Model file for the job. Use its own axes, mm. A direction names the side the tool comes from. Coordinates: 2 decimals unless noted, no trailing zeros. Write each loop counter-clockwise with the first axis right and the second up, starting at its lowest first coordinate (ties: lowest second). Pieces come first, ordered by that corner, then holes.
Q1. Pin check, flat tips, straight feed: P1, Ø2, axis at x = -142, y = 57, coming from the +Z side; P2, Ø16.5, axis at x = -127.5, z = 39.5, coming from the +Y side; P3, Ø16, axis at x = 251, z = -8, coming from the +Y side. Stop position of each tip, or through.
Q2. Pull direction Z, two halves, no side cores. Call faces 1 (the cylindrical face through (205.14, 141.493, 80.832)), 2 (the cylindrical face through (-204.86, 141.314, 81.021)), 3 (the cylindrical face through (205.14, 145.135, 84.259)), 4 (the flat face through (-1, 140, -60)): released by +Z, released by -Z, zero draft, split by the parting line, or undercut.
Q3. Which spindle directions (+Z, -Z, +X, -X, +Y, -Y) get a long thin tool onto all of the face, cutting with end or side? Do faces 5 (the flat face through (195, 142.4, 80)), 6 (the flat face through (-215, 131, 77)), 7 (the flat face through (-250, 125, -20)). Say none if no direction does.
Q4. Drill centre lines: probe 1 along Z at (x, y) = (97, 28); probe 2 along Y at (x, z) = (-201, 77); probe 3 along X at (y, z) = (100, -9). Where is each one in solid material? Low to high.
Q5. Band-saw the part on A-A, the plane y = 57. Write the cut outline in (x, z), plus the area to 3 significant figures.
Q6. Band-saw the part on B-B, the plane x = 74. Write the cut outline in (y, z), plus the area to 3 significant figures.
from build123d import *

# Parameters (mm, degrees)
SKETCH_1_W          = 520
SKETCH_1_H          = 150
EXTRUDE_1_DEPTH     = 140
SKETCH_2_W          = 480
SKETCH_2_H          = 110
CUT_EXTRUDE_1_DEPTH = 120
SKETCH_4_W          = 40
SKETCH_4_H          = 30
EXTRUDE_2_DEPTH     = 30
SKETCH_5_W          = 40
SKETCH_5_H          = 30
EXTRUDE_3_DEPTH     = 30
SKETCH_7_R          = 10
SKETCH_7_R_2        = 5
EXTRUDE_1_2_DEPTH   = 20
EXTRUDE_START       = -20
SKETCH_9_R          = 10
SKETCH_9_R_2        = 5
EXTRUDE_2_2_DEPTH   = 20
SKETCH_11_W         = 40
SKETCH_11_H         = 30
CUT_EXTRUDE_3_DEPTH = 548.622704745
SKETCH_13_W         = 520
SKETCH_13_H         = 150
EXTRUDE_6_DEPTH     = 30
SKETCH_14_W         = 40
SKETCH_14_H         = 5
CUT_EXTRUDE_6_DEPTH = 30
SKETCH_15_W         = 40
SKETCH_15_H         = 5
CUT_EXTRUDE_7_DEPTH = 30
SKETCH_18_W         = 30
SKETCH_18_H         = 15.352958973
CUT_EXTRUDE_8_DEPTH = 30
FILLET_1_R          = 10


with BuildPart() as part:
    # 草圖1 → Extrude 1 (new body)
    with BuildSketch(Plane(origin=(0, 0, 0), x_dir=(1, 0, 0), z_dir=(0, 1, 0))):
        Rectangle(SKETCH_1_W, SKETCH_1_H)
    extrude(amount=EXTRUDE_1_DEPTH)

    # 草圖2 → 除料-伸長1 (cut)
    with BuildSketch(Plane(origin=(0, 140, 0), x_dir=(1, 0, 0), z_dir=(0, 1, 0))):
        Rectangle(SKETCH_2_W, SKETCH_2_H)
    extrude(amount=-CUT_EXTRUDE_1_DEPTH, mode=Mode.SUBTRACT)

    # 草圖4 → Extrude 2 (add)
    with BuildSketch(Plane.XY.offset(80)):
        with Locations((-195, 120)):
            Rectangle(SKETCH_4_W, SKETCH_4_H)
    extrude(amount=-EXTRUDE_2_DEPTH)

    # 草圖5 → 填料-伸長3 (add)
    with BuildSketch(Plane.XY.offset(80)):
        with Locations((195, 120)):
            Rectangle(SKETCH_5_W, SKETCH_5_H)
    extrude(amount=-EXTRUDE_3_DEPTH)

    # 草圖7 → Extrude 1 2 (add)
    with BuildSketch(Plane(origin=(215, 0, 0), x_dir=(0, 0, -1), z_dir=(1, 0, 0))):
        with Locations((-77.5, 137.764599119)):
            Circle(SKETCH_7_R)
        with Locations((-77.5, 137.764599119)):
            Circle(SKETCH_7_R_2, mode=Mode.SUBTRACT)
    extrude(amount=-EXTRUDE_1_2_DEPTH)

    # 草圖9 → Extrude 2 2 (add)
    with BuildSketch(Plane.ZY.offset(215).offset(EXTRUDE_START)):
        with Locations((77.5, 137.764599119)):
            Circle(SKETCH_9_R)
        with Locations((77.5, 137.764599119)):
            Circle(SKETCH_9_R_2, mode=Mode.SUBTRACT)
    extrude(amount=EXTRUDE_2_2_DEPTH)

    # 草圖11 → 除料-伸長3 (cut, through all)
    with BuildSketch(Plane.ZY.offset(260)):
        with Locations((0, 125)):
            Rectangle(SKETCH_11_W, SKETCH_11_H)
    extrude(amount=-CUT_EXTRUDE_3_DEPTH, mode=Mode.SUBTRACT)

    # 草圖13 → 填料-伸長6 (add)
    with BuildSketch(Plane.XZ):
        Rectangle(SKETCH_13_W, SKETCH_13_H)
    extrude(amount=EXTRUDE_6_DEPTH)

    # 草圖14 → 除料-伸長6 (cut)
    with BuildSketch(Plane(origin=(0, 135, 0), x_dir=(1, 0, 0), z_dir=(0, 1, 0))):
        with Locations((195, -52.5)):
            Rectangle(SKETCH_14_W, SKETCH_14_H)
    extrude(amount=-CUT_EXTRUDE_6_DEPTH, mode=Mode.SUBTRACT)

    # 草圖15 → 除料-伸長7 (cut)
    with BuildSketch(Plane(origin=(0, 135, 0), x_dir=(1, 0, 0), z_dir=(0, 1, 0))):
        with Locations((-195, -52.5)):
            Rectangle(SKETCH_15_W, SKETCH_15_H)
    extrude(amount=-CUT_EXTRUDE_7_DEPTH, mode=Mode.SUBTRACT)

    # 草圖18 → 除料-伸長8 (cut)
    with BuildSketch(Plane(origin=(0, 0, -75), x_dir=(-1, 0, 0), z_dir=(0, 0, -1))):
        with Locations((0, 122.323520514)):
            Rectangle(SKETCH_18_W, SKETCH_18_H)
    extrude(amount=-CUT_EXTRUDE_8_DEPTH, mode=Mode.SUBTRACT)

    # 圓角1
    fillet_1_edges = [part.edges().sort_by_distance(p)[0] for p in [
        (0, 130, -75),
    ]]
    fillet(fillet_1_edges, radius=FILLET_1_R - 0.0001)  # a hair under: the kernel refuses the full size


solid = part.part
Answer sheet:
1. P1: stops at z = 75
1. P2: stops at y = 20
1. P3: stops at y = 110
2. face 1: undercut
2. face 2: undercut
2. face 3: split by the parting line
2. face 4: zero draft
3. face 5: +Z, +Y
3. face 6: +Z, -X, +Y
3. face 7: +X, -X, +Y
4. probe 1: z = -75 to -55, 55 to 75
4. probe 2: y = 105 to 135, 142.74 to 147.75
4. probe 3: x = -260 to -240, 240 to 260
5. outline: (-260, -75) - (260, -75) - (260, 75) - (-260, 75) - close; hole (-240, -55) - (240, -55) - (240, 55) - (-240, 55) - close
5. area: 25,200 mm2
6. outline: (-30, -75) - (140, -75) - (140, -55) - (20, -55) - (20, 55) - (140, 55) - (140, 75) - (-30, 75) - close
6. area: 12,300 mm2
